Autodesk Inventor part; units mm, degrees
ref_plane "YZ Plane" through (0, 0, 0) normal (1, 0, 0) x (0, 1, 0)
ref_plane "XZ Plane" through (0, 0, 0) normal (0, 1, 0) x (-1, 0, 0)
ref_plane "XY Plane" through (0, 0, 0) normal (0, 0, 1) x (1, 0, 0)
sketch "Sketch1" plane through (0, 0, 0) normal (0, 1, 0) x (-1, 0, 0)
  circle A0 centre (0, 0) radius 21.5
  dimension "d1" = 43
extrude "Extrusion1" add sketch "Sketch1" along normal blind 3
sketch "Sketch2" plane through (0, 3, 0) normal (0, 1, 0) x (1, 0, 0)
  arc A0 (15.6228, -13.2732) -> (-15.6228, -13.2732) centre (0, 0) ccw
  arc A1 (16.9137, -13.2732) -> (-16.9137, -13.2732) centre (0, 0) ccw
  circle A2 centre (0, 0) radius 21.5
  line L0 (-16.9137, -13.2732) -> (-15.6228, -13.2732)
  line L1 (15.6228, -13.2732) -> (16.9137, -13.2732)
  dimension "d4" = 41
extrude "Extrusion2" add sketch "Sketch2" along normal blind 3 contours A0 L0 A1 L1
sketch "Sketch3" plane through (0, 3, 0) normal (0, 1, 0) x (1, 0, 0)
  circle A0 centre (-10, 0) radius 3
  circle A1 centre (10, 0) radius 3
  point P0 (0, 0)
  dimension "d7" = 6
  dimension "d8" = 6
extrude "Extrusion3" cut sketch "Sketch3" against normal blind 10 contours A0
sketch "Sketch4" plane through (0, 3, 0) normal (0, 1, 0) x (1, 0, 0)
  circle A0 centre (10, 0) radius 3
  point P0 (0, 0)
  dimension "d11" = 6
extrude "Extrusion4" cut sketch "Sketch4" against normal blind 10
sketch "Sketch5" plane through (0, 3, 0) normal (0, 1, 0) x (1, 0, 0)
  line L0 (0, 6) -> (5, 6)
  line L1 (5, 6) -> (5, -6)
  line L2 (5, -6) -> (-5, -6)
  line L3 (-5, -6) -> (-5, 6)
  line L4 (-5, 6) -> (0, 6)
  point P0 (0, 0)
extrude "Extrusion5" cut sketch "Sketch5" against normal blind 10
sketch "Sketch6" plane through (0, 3, 0) normal (0, 1, 0) x (1, 0, 0)
  line L0 (5, 6) -> (5.7071, 6.7071)
  line L1 (5, 6) -> (6, 6) construction
  line L2 (5.7071, 6.7071) -> (5.7071, -7.2929)
  line L3 (5.7071, -7.2929) -> (-5.7269, -7.2929)
  line L4 (-5.7269, -7.2929) -> (-5.7269, 6.7071)
  line L5 (-5.7269, 6.7071) -> (5.7071, 6.7071)
  point P0 (0, 0)
  dimension "d21" = 1
  dimension "d22" = 45
  dimension "d23" = 14
  dimension "d24" = 45
extrude "Extrusion6" cut sketch "Sketch6" against normal blind 10
properties part number "EndCapProper"
Part model, mm, in its own coordinate system. A direction names the side the tool comes from. Give positions to 0.01 mm unless a question says otherwise; leave off trailing zeros. Order: outer loops, then holes, each group sorted by start corner. A loop starts at its lowest first (then second) coordinate and runs counter-clockwise, first axis right, second up. Notation, with made-up numbers: (-24, 13) - (28, 13) arc R11 cw to (28, 24) - close; hole circle Ø2 at (64, 7). An arc over 180 degrees is marked (long way). Use one line per item in the form item = value.
Item 1: Pin check, flat tips, straight feed: pin 1 Ø3 at (x, y) = (11.5, 4) entering from +Z; pin 2 Ø2 at (x, y) = (-2, 3) entering from +Z; pin 3 Ø8 at (x, z) = (8.5, 8.5) entering from -Y; pin 4 Ø20.5 at (x, z) = (0, -6.5) entering from +Y. Stop position of each tip, or through.
Solution:
pin_1 = 18.83
pin_2 = 21.48
pin_3 = 0
pin_4 = 3
Item 2: Slice it at B-B on x = -10. Give the cut face in (y, z), and give its area (3 significant figures).
Solution:
outline = (0, -19.03) - (6, -19.03) - (6, -17.9) - (3, -17.9) - (3, -3) - (0, -3) - close; (0, 3) - (3, 3) - (3, 19.03) - (0, 19.03) - close
area = 99.6 mm2
Item 3: Probe probe 1 along X at (y, z) = (2.45, 0); probe 2 along X at (y, z) = (3.75, 0); probe 3 along X at (y, z) = (0.4, 1). List the from-to ranges inside material, lowest first. Write a range as from..to.
Solution:
probe_1 = -21.5..-13, -7..-5.73, 5.71..7, 13..21.5
probe_2 = -21.5..-20.5, 20.5..21.5
probe_3 = -21.48..-12.83, -7.17..-5.73, 5.71..7.17, 12.83..21.48
Item 4: Two-plate mould, pull along Z, no slides. Class faces 1 (the face through (2.799, 1.479, -21.317)), 2 (the face through (0, 0, -9)), 3 (the face through (-5.727, 2, 0)): released by +Z, released by -Z, zero draft, split by the parting line, or undercut.
Solution:
face_1 = split by the parting line
face_2 = zero draft
face_3 = undercut
Item 5: Slice it at D-D on x = -1. Give the cut face in (y, z), and give its area (3 significant figures).
Solution:
outline = (0, -21.48) - (6, -21.48) - (6, -20.48) - (3, -20.48) - (3, -6.71) - (0, -6.71) - close; (0, 7.29) - (3, 7.29) - (3, 21.48) - (0, 21.48) - close
area = 89.9 mm2
Item 6: Slice it at C-C on y = 0.8. Give the cut face in (x, z).
Solution:
outline = circle Ø43 at (0, 0); hole circle Ø6 at (-10, 0); hole (-5.73, -6.71) - (5.71, -6.71) - (5.71, 7.29) - (-5.73, 7.29) - close; hole circle Ø6 at (10, 0)
Item 7: Which spindle directions (+Z, -Z, +X, -X, +Y, -Y) get a long thin tool onto all of the face, cutting with end or side? Do faces 4 (the face through (5.707, 2, 0)), 5 (the face through (-16, 4, 13.273)), 6 (the face through (-0.65, 4.48, -20.49)). Say none if no direction does.
Solution:
face_4 = +Y, -Y
face_5 = +Z, +X, -X, +Y
face_6 = +Y
Item 8: Slice it at A-A on z = 0. Give the cut face in (x, y), and give its area (3 significant figures).
Solution:
outline = (-21.5, 0) - (-13, 0) - (-13, 3) - (-20.5, 3) - (-20.5, 6) - (-21.5, 6) - close; (-7, 0) - (-5.73, 0) - (-5.73, 3) - (-7, 3) - close; (5.71, 0) - (7, 0) - (7, 3) - (5.71, 3) - close; (13, 0) - (21.5, 0) - (21.5, 6) - (20.5, 6) - (20.5, 3) - (13, 3) - close
area = 64.7 mm2
